Input: part model. Units: mm. Frame: model coordinates. A direction names the side the tool comes from. Round coordinates to 2 decimals unless told otherwise and drop trailing zeros. Loops run counter-clockwise (first coordinate to the right, second up) from the corner with the lowest first, then second, coordinate; pieces in that order, holes last. Notation, with made-up numbers: M -10,37 L 28,37 A20 ccw 28,59 Z; hole C 6,14.25 d8. An arc over 180 degrees is marked long. Put each result on its own line as item: value. Start each with the question number.
1) Pin query (flat end, axial travel): pin 1 (0.9 mm diameter, centred on x = 18.5, y = -1.5, fed in from -Z); pin 2 (16 mm diameter, centred on x = 7.5, y = -1.5, fed in from +Z); pin 3 (3.5 mm diameter, centred on y = 0, z = 4.76, fed in from -X); pin 4 (7 mm diameter, centred on x = 0, y = 0, fed in from +Z). Return the tip coordinate at first contact, or that it passes through.
2) Line query: probe 1 along Y at (x, z) = (-18.65, 15.5); probe 2 along Y at (x, z) = (0, 5.5); probe 3 along X at (y, z) = (19, 21.5). Output: solid intervals per line, ascending.
3) Section C-C on y = 0. State how many separate pieces and enclosed holes the cut face has, plus the area to 3 significant figures.
4) Section B-B on z = 18.75. Output: boundary loops of the cut face in (x, y).
5) Draft query along X for faces 1 (the face through (-28, 0, 12)), 2 (the face through (-19.28, 19.65, 11.91)), 3 (the face through (28, 0, 12)), 4 (the face through (-19.28, -19.65, 11.91)). Return one class per face: +X half, -X half, draft (parallel to the pull), parting line (faces both ways), or undercut.
6) Reachability of faces 5 (the face through (-23.756, 0.087, 6.745)), 6 (the face through (11.83, 17.32, 17.18)), 7 (the face through (-3.441, -15.497, 22.498)), 8 (the face through (-18.449, 1.984, 5.898)) from +Z, -Z, +X, -X, +Y, -Y: full face, straight path, thin tool, end or side. Return the list, or none.
7) Section A-A on x = 0. Output: boundary loops of the cut face in (y, z) (3 decimals), plus the area to 3 significant figures.
8) Section D-D on z = 8.25. Output: boundary loops of the cut face in (x, y), plus the area to 3 significant figures.
from build123d import *

# Parameters (mm, degrees)
SKETCH1_W               = 56
SKETCH1_H               = 51.5
BOSS_EXTRUDE1_DEPTH     = 23.5
SKETCH2_R               = 15.875
CUT_EXTRUDE1_DEPTH      = 2.032
SKETCH3_R               = 12.7
CUT_EXTRUDE2_DEPTH      = 10.668
SKETCH4_R               = 3.8354
CUT_EXTRUDE3_DEPTH      = 11.8
SKETCH5_R               = 6.35
CUT_EXTRUDE4_DEPTH      = 2.794
SKETCH6_R               = 4.2164
CUT_EXTRUDE5_DEPTH      = 25.4
SKETCH7_R               = 1.984375
CUT_EXTRUDE6_DEPTH      = 6.35
SKETCH8_R               = 1.984375
CUT_EXTRUDE7_DEPTH      = 11.1125
SKETCH9_R               = 1.1811
CUT_EXTRUDE8_DEPTH      = 24.5
MIRROR4_COPY_1_SKETCH_R = 1.1811
MIRROR4_COPY_1_DEPTH    = 24.5


with BuildPart() as part:
    # Sketch1 → Boss-Extrude1 (new body)
    with BuildSketch(Plane.XY):
        Rectangle(SKETCH1_W, SKETCH1_H)
    extrude(amount=BOSS_EXTRUDE1_DEPTH)

    # Sketch2 → Cut-Extrude1 (cut)
    with BuildSketch(Plane.XY.offset(23.5)):
        Circle(SKETCH2_R)
    extrude(amount=-CUT_EXTRUDE1_DEPTH, mode=Mode.SUBTRACT)

    # Sketch3 → Cut-Extrude2 (cut)
    with BuildSketch(Plane.XY.offset(21.468)):
        Circle(SKETCH3_R)
    extrude(amount=-CUT_EXTRUDE2_DEPTH, mode=Mode.SUBTRACT)

    # Sketch4 → Cut-Extrude3 (cut, through all)
    with BuildSketch(Plane.XY.offset(10.8)):
        Circle(SKETCH4_R)
    extrude(amount=-CUT_EXTRUDE3_DEPTH, mode=Mode.SUBTRACT)

    # Sketch5 → Cut-Extrude4 (cut)
    with BuildSketch(Plane(origin=(0, 0, 0), x_dir=(-1, 0, 0), z_dir=(0, 0, -1))):
        Circle(SKETCH5_R)
    extrude(amount=-CUT_EXTRUDE4_DEPTH, mode=Mode.SUBTRACT)

    # Sketch6 → Cut-Extrude5 (cut)
    with BuildSketch(Plane(origin=(0, 25.75, 0), x_dir=(1, 0, 0), z_dir=(0, 1, 0))):
        with Locations((7.9375, -15.5625)):
            Circle(SKETCH6_R)
    extrude(amount=-CUT_EXTRUDE5_DEPTH, mode=Mode.SUBTRACT)

    # Sketch7 → Cut-Extrude6 (cut)
    with BuildSketch(Plane(origin=(0, 0, 0), x_dir=(-1, 0, 0), z_dir=(0, 0, -1))):
        with Locations((-18.475, 0)):
            Circle(SKETCH7_R)
    cut_extrude6 = extrude(amount=-CUT_EXTRUDE6_DEPTH, mode=Mode.SUBTRACT)

    # Mirror1: Cut-Extrude6 across plane
    add(cut_extrude6.mirror(Plane(origin=(0, 0, 0), x_dir=(0, 0, 1), z_dir=(1, 0, 0))), mode=Mode.SUBTRACT)

    # Sketch8 → Cut-Extrude7 (cut)
    with BuildSketch(Plane(origin=(28, 0, 0), x_dir=(0, 0, -1), z_dir=(1, 0, 0))):
        with Locations((-4.7625, 0)):
            Circle(SKETCH8_R)
    cut_extrude7 = extrude(amount=-CUT_EXTRUDE7_DEPTH, mode=Mode.SUBTRACT)

    # Mirror2: Cut-Extrude7 across plane
    add(cut_extrude7.mirror(Plane(origin=(0, 0, 0), x_dir=(0, 0, 1), z_dir=(1, 0, 0))), mode=Mode.SUBTRACT)

    # Sketch9 → Cut-Extrude8 (cut, through all)
    with BuildSketch(Plane.XY.offset(23.5)):
        with Locations((18.65, 18.65)):
            Circle(SKETCH9_R)
    cut_extrude8 = extrude(amount=-CUT_EXTRUDE8_DEPTH, mode=Mode.SUBTRACT)

    # Mirror3: Cut-Extrude8 across plane
    add(cut_extrude8.mirror(Plane.ZX), mode=Mode.SUBTRACT)

    # Mirror4: Cut-Extrude8 across plane
    add(cut_extrude8.mirror(Plane(origin=(0, 0, 0), x_dir=(0, 0, 1), z_dir=(1, 0, 0))), mode=Mode.SUBTRACT)

    # Mirror4 copy 1 sketch → Mirror4 copy 1 (cut, through all)
    with BuildSketch(Plane(origin=(0, 0, 23.5), x_dir=(-1, 0, 0), z_dir=(0, 0, 1))):
        with Locations((18.65, 18.65)):
            Circle(MIRROR4_COPY_1_SKETCH_R)
    extrude(amount=-MIRROR4_COPY_1_DEPTH, mode=Mode.SUBTRACT)


solid = part.part
Geometry results:
1. pin 1: stops at z = 6.35
1. pin 2: stops at z = 21.47
1. pin 3: stops at x = -16.89
1. pin 4: passes through
2. probe 1: y = -25.75 to -19.83, -17.47 to 17.47, 19.83 to 25.75
2. probe 2: y = -25.75 to -3.84, 3.84 to 25.75
2. probe 3: x = -28 to -19.78, -17.52 to 17.52, 19.78 to 28
3. separate pieces: 4
3. enclosed holes: 0
3. area: 771 mm²
4. outline: M -28,-25.75 L 28,-25.75 L 28,25.75 L 10.7,25.75 L 10.7,6.84 A12.7 cw long 5.18,11.6 L 5.18,25.75 L -28,25.75 Z; hole C -18.65,-18.65 d2.36; hole C -18.65,18.65 d2.36; hole C 18.65,-18.65 d2.36; hole C 18.65,18.65 d2.36
5. face 1: -X half
5. face 2: undercut
5. face 3: +X half
5. face 4: undercut
6. face 5: -X
6. face 6: +Y
6. face 7: +Z
6. face 8: -Z
7. outline: M -25.75,0 L -6.35,0 L -6.35,2.794 L -3.835,2.794 L -3.835,10.8 L -12.7,10.8 L -12.7,21.468 L -15.875,21.468 L -15.875,23.5 L -25.75,23.5 Z; M 3.835,2.794 L 6.35,2.794 L 6.35,0 L 25.75,0 L 25.75,23.5 L 15.875,23.5 L 15.875,21.468 L 12.7,21.468 L 12.7,10.8 L 3.835,10.8 Z
7. area: 778 mm²
8. outline: M -28,-25.75 L 28,-25.75 L 28,25.75 L -28,25.75 Z; hole C -18.65,-18.65 d2.36; hole C -18.65,18.65 d2.36; hole C 0,0 d7.67; hole C 18.65,-18.65 d2.36; hole C 18.65,18.65 d2.36
8. area: 2,820 mm²
